from build123d import *

# Parameters (mm, degrees)
SKETCH1_W               = 13.42
SKETCH1_H               = 12.6
BOSS_EXTRUDE1_DEPTH     = 6.5
CUT_EXTRUDE1_DEPTH      = 18.598695974
CUT_EXTRUDE1_DEPTH_BACK = 18.598695974
SKETCH4_W               = 1.5
SKETCH4_H               = 7


with BuildPart() as part:
    # Sketch1 → Boss-Extrude1 (new body)
    with BuildSketch(Plane.XY):
        Rectangle(SKETCH1_W, SKETCH1_H)
    extrude(amount=BOSS_EXTRUDE1_DEPTH)

    # Sketch3 → Revolve1 (revolve)
    with BuildSketch(Plane(origin=(0, 0, 0), x_dir=(1, 0, 0), z_dir=(0, 1, 0))):
        Polygon((0, 0), (3.5, 0), (3.5, 5), (2.063862247, 5), (2.063862247, 5.599280985), (3, 5.599280985), (3, 15), (0, 15), align=None)
    revolve(axis=Axis((0, 0, 0), (0, 0, -1)))

    # Sketch4 → Cut-Extrude1 (cut, two sides: drawn at the far end of the back side and taken through both)
    with BuildSketch(Plane(origin=(0, 0, 0), x_dir=(1, 0, 0), z_dir=(0, 1, 0)).offset(-CUT_EXTRUDE1_DEPTH_BACK)):
        with Locations((2.25, 11.5)):
            Rectangle(SKETCH4_W, SKETCH4_H)
    extrude(amount=CUT_EXTRUDE1_DEPTH + CUT_EXTRUDE1_DEPTH_BACK, mode=Mode.SUBTRACT)


solid = part.part
CAD build for the part. Positions are in the model's coordinates, mm. A direction names the side the tool comes from. Coordinates: 2 decimals unless noted, no trailing zeros. Loops run counter-clockwise (first coordinate to the right, second up) from the corner with the lowest first, then second, coordinate; pieces in that order, holes last. Notation, with made-up numbers: (24.25, -1.5) -> (67.25, -1.5) arc R12 ccw to (67.25, 11.5) -> close; hole circle Ø1 at (89, 72.25). An arc over 180 degrees is marked (long way). One line per item, written item: value.
1. Drill centre lines: line 1 (Z direction, x = 2, y = 2); line 2 (Z direction, x = 3, y = 4.5); line 3 (Z direction, x = -3.25, y = -1). Where is each one in solid material? Low to high. Write a range as [from, to].
Answers:
line 1: z = [-8, -5.6], [-5, 6.5]
line 2: z = [0, 6.5]
line 3: z = [-5, 6.5]
2. Pull direction Z, two halves, no side cores. Call faces 4 (the face through (2, 2, -5)), 5 (the face through (-6.71, 0, 3)), 6 (the face through (2, 0, -8)): pulls with the +Z half, pulls with the -Z half, needs draft (parallel to the pull), parting line crosses it, or undercut.
Answers:
face 4: undercut
face 5: needs draft
face 6: pulls with the -Z half
3. Slice it at A-A on y = 0. Write the cut outline in (x, z), and give its area (3 significant figures).
Answers:
outline: (-6.71, 0) -> (-3.5, 0) -> (-3.5, -5) -> (-2.06, -5) -> (-2.06, -5.6) -> (-3, -5.6) -> (-3, -15) -> (1.5, -15) -> (1.5, -8) -> (3, -8) -> (3, -5.6) -> (2.06, -5.6) -> (2.06, -5) -> (3.5, -5) -> (3.5, 0) -> (6.71, 0) -> (6.71, 6.5) -> (-6.71, 6.5) -> close
area: 171 mm^2
4. Slice it at D-D on z = -7.5. Write the cut outline in (x, y).
Answers:
outline: circle Ø6 at (0, 0)
5. Slice it at B-B on x = 0. Write the cut outline in (y, z), and give its area (3 significant figures).
Answers:
outline: (-6.3, 0) -> (-3.5, 0) -> (-3.5, -5) -> (-2.06, -5) -> (-2.06, -5.6) -> (-3, -5.6) -> (-3, -15) -> (3, -15) -> (3, -5.6) -> (2.06, -5.6) -> (2.06, -5) -> (3.5, -5) -> (3.5, 0) -> (6.3, 0) -> (6.3, 6.5) -> (-6.3, 6.5) -> close
area: 176 mm^2
6. Flat gauge pins, fed straight in: P1, Ø4, axis at y = -1, z = -13, coming from the +X side; P2, Ø1.5, axis at x = 4, y = -3, coming from the -Z side; P3, Ø1.7, axis at x = 2.5, y = -1, coming from the -Z side. Where does each tip first touch, or does it go through?
Answers:
P1: stops at x = 1.5
P2: stops at z = 0
P3: stops at z = -8
7. Slice it at C-C on x = 2.75. Write the cut outline in (y, z), and give its area (3 significant figures).
Answers:
outline: (-6.3, 0) -> (-2.17, 0) -> (-2.17, -5) -> (2.17, -5) -> (2.17, 0) -> (6.3, 0) -> (6.3, 6.5) -> (-6.3, 6.5) -> close; (-1.2, -8) -> (1.2, -8) -> (1.2, -5.6) -> (-1.2, -5.6) -> close
area: 109 mm^2
8. Which spindle directions (+Z, -Z, +X, -X, +Y, -Y) get a long thin tool onto all of the face, cutting with end or side? Do faces 1 (the face through (-0.447, 2.015, -5.304)), 2 (the face through (3.233, 1.341, -2.535)), 3 (the face through (1.5, 0, -11)). Say none if no direction does.
Answers:
face 1: none
face 2: -Z
face 3: -Z, +X, +Y, -Y
